```python
from build123d import *

# Parameters (mm, degrees)
F0_W     = 730.25
F0_H     = 495.3
F1_DEPTH = 977.9
F2_W     = 692.15
F2_H     = 495.3
F3_DEPTH = 25.4
F4_W     = 692.15
F4_H     = 914.4
F5_DEPTH = 469.9
F6_W     = 19.05
F6_H     = 914.4
F7_DEPTH = 469.9
F8_W     = 50.8
F8_H     = 50.8
F9_DEPTH = 50.8
F10_R    = 5.08
F11_R    = 5.08
F12_R    = 5.08
F13_R    = 5.08


with BuildPart() as f1:
    # F0 (on Top) → F1 (new body)
    with BuildSketch(Plane.XY):
        Rectangle(F0_W, F0_H)
    extrude(amount=F1_DEPTH)

    # F2 (on face) → F3 (cut)
    with BuildSketch(Plane.XY.offset(977.9)):
        Rectangle(F2_W, F2_H)
    extrude(amount=-F3_DEPTH, mode=Mode.SUBTRACT)

    # F4 (on face) → F5 (cut)
    with BuildSketch(Plane.XZ.offset(247.65)):
        with Locations((0, 476.25)):
            Rectangle(F4_W, F4_H)
    extrude(amount=-F5_DEPTH, mode=Mode.SUBTRACT)

    # F6 (on face) → F7 (join)
    with BuildSketch(Plane.XZ.offset(-222.25)):
        with Locations((0, 476.25)):
            Rectangle(F6_W, F6_H)
    extrude(amount=F7_DEPTH)

    # F8 (on face) → F9 (join)
    with BuildSketch(Plane(origin=(0, 0, 0), x_dir=(1, 0, 0), z_dir=(0, 0, -1))):
        with Locations((288.925, 222.25)):
            Rectangle(F8_W, F8_H)
        with Locations((288.925, -222.25)):
            Rectangle(F8_W, F8_H)
        with Locations((-288.925, -222.25)):
            Rectangle(F8_W, F8_H)
        with Locations((-288.925, 222.25)):
            Rectangle(F8_W, F8_H)
    extrude(amount=F9_DEPTH)

    # F10
    f10_edges = [f1.edges().sort_by_distance(p)[0] for p in [
        (-263.525, -222.25, -50.8),
        (-288.925, -196.85, -50.8),
        (-288.925, -247.65, -50.8),
        (-314.325, -222.25, -50.8),
        (-314.325, 222.25, -50.8),
        (-288.925, 196.85, -50.8),
        (-263.525, 222.25, -50.8),
        (-288.925, 247.65, -50.8),
    ]]
    fillet(f10_edges, radius=F10_R)

    # F11
    f11_edges = [f1.edges().sort_by_distance(p)[0] for p in [
        (314.325, -222.25, -50.8),
        (288.925, -247.65, -50.8),
        (263.525, -222.25, -50.8),
        (288.925, -196.85, -50.8),
    ]]
    fillet(f11_edges, radius=F11_R)

    # F12
    f12_edges = [f1.edges().sort_by_distance(p)[0] for p in [
        (288.925, 247.65, -50.8),
        (314.325, 222.25, -50.8),
        (288.925, 196.85, -50.8),
        (263.525, 222.25, -50.8),
    ]]
    fillet(f12_edges, radius=F12_R)

    # F13
    f13_edges = [f1.edges().sort_by_distance(p)[0] for p in [
        (355.6, -247.65, 977.9),
        (-355.6, -247.65, 977.9),
        (355.6, 247.65, 977.9),
        (-355.6, 247.65, 977.9),
    ]]
    fillet(f13_edges, radius=F13_R)


solid = f1.part
```
For this review, take the finished solid that the model builds, in its own axes (mm). A direction names the side the tool comes from. Round coordinates to 2 decimals unless told otherwise and drop trailing zeros. Order: outer loops, then holes, each group sorted by start corner. A loop starts at its lowest first (then second) coordinate and runs counter-clockwise, first axis right, second up. Notation, with made-up numbers: (-14.5, -22.75) -> (29.5, -22.75) arc R27 ccw to (29.5, -0.75) -> close; hole circle Ø6 at (-26.75, 28). An arc over 180 degrees is marked (long way). Use a Markdown table: item, result.
Item 1: Take a section at C-C (z = 342). State the section outline as (x, y) points (3 decimals), plus the area to 3 significant figures.
Resolved:
| item | result |
|---|---|
| outline | (-365.125, -247.65) -> (-346.075, -247.65) -> (-346.075, 222.25) -> (-9.525, 222.25) -> (-9.525, -247.65) -> (9.525, -247.65) -> (9.525, 222.25) -> (346.075, 222.25) -> (346.075, -247.65) -> (365.125, -247.65) -> (365.125, 247.65) -> (-365.125, 247.65) -> close |
| area | 45,400 mm² |
Item 2: Take a section at D-D (x = -291). State the section outline as (y, z) points, plus the area to 3 significant figures.
Resolved:
| item | result |
|---|---|
| outline | (-247.65, -45.72) arc R5.08 ccw to (-242.57, -50.8) -> (-201.93, -50.8) arc R5.08 ccw to (-196.85, -45.72) -> (-196.85, 0) -> (196.85, 0) -> (196.85, -45.72) arc R5.08 ccw to (201.93, -50.8) -> (242.57, -50.8) arc R5.08 ccw to (247.65, -45.72) -> (247.65, 952.5) -> (-247.65, 952.5) -> (-247.65, 933.45) -> (222.25, 933.45) -> (222.25, 19.05) -> (-247.65, 19.05) -> close |
| area | 47,200 mm² |
Item 3: For line 1 along X through (y, z) = (-128, 370.5) (3 decimals); line 2 along Z through (x, y) = (-47, -91); line 3 along Y through (x, z) = (35, 21.5), list the stretches that pass through material, from the lowest coordinate up. Write a range as [from, to].
Resolved:
| item | result |
|---|---|
| line 1 | x = [-365.125, -346.075], [-9.525, 9.525], [346.075, 365.125] |
| line 2 | z = [0, 19.05], [933.45, 952.5] |
| line 3 | y = [222.25, 247.65] |
Item 4: Take a section at A-A (y = 36.5). State the section outline as (x, z) points (3 decimals).
Resolved:
| item | result |
|---|---|
| outline | (-365.125, 0) -> (365.125, 0) -> (365.125, 977.9) -> (346.075, 977.9) -> (346.075, 952.5) -> (-346.075, 952.5) -> (-346.075, 977.9) -> (-365.125, 977.9) -> close; hole (-346.075, 19.05) -> (-9.525, 19.05) -> (-9.525, 933.45) -> (-346.075, 933.45) -> close; hole (9.525, 19.05) -> (346.075, 19.05) -> (346.075, 933.45) -> (9.525, 933.45) -> close |
Item 5: Take a section at B-B (x = 247). State the section outline as (y, z) points.
Resolved:
| item | result |
|---|---|
| outline | (-247.65, 0) -> (247.65, 0) -> (247.65, 952.5) -> (-247.65, 952.5) -> (-247.65, 933.45) -> (222.25, 933.45) -> (222.25, 19.05) -> (-247.65, 19.05) -> close |
Item 6: Machinability: for faces 4 (the flat face through (346.075, -3, 965)), 5 (the flat face through (314.325, 223, -23)), 6 (the flat face through (-180, 222.25, 483)), 7 (the flat face through (289, -196.85, -23)), which of the approach directions +Z, -Z, +X, -X, +Y, -Y give a long, thin tool a straight path to every point of the face, cutting with its end or side? Answer none if there is none.
Resolved:
| item | result |
|---|---|
| face 4 | +Z, +Y, -Y |
| face 5 | -Z, +X, +Y, -Y |
| face 6 | -Y |
| face 7 | -Z, +X, -X |
Item 7: For pin 1 (3 mm diameter, centred on x = -135.5, y = -189, fed in from +Z); pin 2 (12 mm diameter, centred on x = 247.5, z = 275.5, fed in from -Y); pin 3 (4 mm diameter, centred on x = 0, y = 139.5, fed in from -Z), all flat-tipped, find the tip position at first contact; note any pin that passes through.
Resolved:
| item | result |
|---|---|
| pin 1 | stops at z = 952.5 |
| pin 2 | stops at y = 222.25 |
| pin 3 | stops at z = 0 |
Item 8: Draft analysis for pull direction Z (two halves, no side actions). For faces 1 (the flat face through (-289, -223, -50.8)), 2 (the flat face through (-289, -196.85, -23)), 3 (the flat face through (-9.525, -9, 470)), state which applies: +Z half, -Z half, draft (parallel to the pull), parting line (faces both ways), or undercut.
Resolved:
| item | result |
|---|---|
| face 1 | -Z half |
| face 2 | draft |
| face 3 | undercut |
